Geometry: final body of the model. Coordinates: model frame, mm. A direction names the side the tool comes from. Coordinates: 2 decimals unless noted, no trailing zeros. Loops run counter-clockwise (first coordinate to the right, second up) from the corner with the lowest first, then second, coordinate; pieces in that order, holes last. Notation, with made-up numbers: (-34, 5.5) - (24, 5.5) arc R15 ccw to (24, 24.5) - close; hole circle Ø7 at (28.5, -2). An arc over 180 degrees is marked (long way). Write each question's results on one line, items separated by ' | '. Start each with the question number.
from build123d import *

# Parameters (mm, degrees)
BOSS_EXTRUDE1_DEPTH = 15
SKETCH5_R           = 17
CUT_EXTRUDE3_DEPTH  = 12
SKETCH8_R           = 3.5
CUT_EXTRUDE5_DEPTH  = 3
CUT_EXTRUDE8_DEPTH  = 2
BOSS_EXTRUDE2_DEPTH = 3
BOSS_EXTRUDE3_DEPTH = 3
SKETCH14_R          = 2
SKETCH14_R_2        = 1.65
CUT_EXTRUDE10_DEPTH = 3
SKETCH15_R          = 0.5
SKETCH15_R_2        = 4
SKETCH15_W          = 23.5
SKETCH15_H          = 12.4
CUT_EXTRUDE11_DEPTH = 3
BOSS_EXTRUDE4_DEPTH = 18.1
FILLET2_R           = 5
FILLET3_R           = 1


with BuildPart() as part:
    # Sketch1 → Boss-Extrude1 (new body)
    with BuildSketch(Plane(origin=(0, 0, 0), x_dir=(0, 0, -1), z_dir=(1, 0, 0))):
        with BuildLine():
            Line((0, 20), (80, 20))
            Line((80, 20), (80, -20))
            Line((80, -20), (0, -20))
            ThreePointArc((0, -20), (-20, 0), (0, 20))
        make_face()
    extrude(amount=BOSS_EXTRUDE1_DEPTH)

    # Sketch5 → Cut-Extrude3 (cut)
    with BuildSketch(Plane.ZY):
        Circle(SKETCH5_R)
    extrude(amount=-CUT_EXTRUDE3_DEPTH, mode=Mode.SUBTRACT)

    # Sketch8 → Cut-Extrude5 (cut)
    with BuildSketch(Plane.ZY.offset(-12)):
        Circle(SKETCH8_R)
    extrude(amount=-CUT_EXTRUDE5_DEPTH, mode=Mode.SUBTRACT)

    # Sketch10 → Cut-Extrude8 (cut)
    with BuildSketch(Plane.ZY.offset(-12)):
        with BuildLine():
            Line((-11.740635761, 8.915001197), (-3.490542592, -0.257123349))
            ThreePointArc((-3.490542592, -0.257123349), (-2.474873734, 2.474873734), (0.257123349, 3.490542592))
            Line((0.257123349, 3.490542592), (-8.915001197, 11.740635761))
            ThreePointArc((-8.915001197, 11.740635761), (-11.667842746, 11.667842746), (-11.740635761, 8.915001197))
        make_face()
        with BuildLine():
            Line((11.740635761, -8.915001197), (3.490542592, 0.257123349))
            ThreePointArc((3.490542592, 0.257123349), (3.497634849, 0.12864861), (3.5, 0))
            ThreePointArc((3.5, 0), (2.382233015, -2.564169624), (-0.257123349, -3.490542592))
            Line((-0.257123349, -3.490542592), (8.915001197, -11.740635761))
            ThreePointArc((8.915001197, -11.740635761), (11.667842746, -11.667842746), (11.740635761, -8.915001197))
        make_face()
    extrude(amount=-CUT_EXTRUDE8_DEPTH, mode=Mode.SUBTRACT)

    # Sketch13 → Boss-Extrude3 (add)
    with BuildSketch(Plane(origin=(0, -4.9, 0), x_dir=(1, 0, 0), z_dir=(0, 1, 0))):
        Polygon((-17.5, 80), (32.5, 80), (35.5, 83), (35.5, 103), (30.5, 108), (-15.5, 108), (-20.5, 103), (-20.5, 83), align=None)
    extrude(amount=BOSS_EXTRUDE3_DEPTH)

    # Sketch15 → Cut-Extrude11 (cut)
    with BuildSketch(Plane(origin=(0, -1.9, 0), x_dir=(1, 0, 0), z_dir=(0, 1, 0))):
        with Locations(Location((-16.65, 100, 0), (0, 0, 270))):
            Circle(SKETCH15_R)
        with Locations(Location((11.85, 100, 0), (0, 0, 270))):
            Circle(SKETCH15_R)
        with Locations(Location((22.5, 100, 0), (0, 0, 270))):
            Circle(SKETCH15_R_2)
        with Locations((-2.4, 100)):
            Rectangle(SKETCH15_W, SKETCH15_H)
    extrude(amount=-CUT_EXTRUDE11_DEPTH, mode=Mode.SUBTRACT)



with BuildPart() as body_2:
    # Sketch12 → Boss-Extrude2 (new body)
    with BuildSketch(Plane.XZ.offset(20)):
        Polygon((-17.5, -80), (32.5, -80), (37.5, -85), (37.5, -105), (22, -120.5), (22, -125), (17, -130), (-2, -130), (-7, -125), (-7, -120.5), (-22.5, -105), (-22.5, -85), align=None)
    extrude(amount=-BOSS_EXTRUDE2_DEPTH)

    # Sketch14 → Cut-Extrude10 (cut)
    with BuildSketch(Plane.XZ.offset(20)):
        with Locations(Location((-7.5, -100, 0), (0, 0, 270))):
            Circle(SKETCH14_R)
        with Locations(Location((22.5, -100, 0), (0, 0, 270))):
            Circle(SKETCH14_R_2)
        with Locations(Location((15, -123, 0), (0, 0, 270))):
            Circle(SKETCH14_R_2)
        with Locations(Location((0, -123, 0), (0, 0, 270))):
            Circle(SKETCH14_R_2)
    extrude(amount=-CUT_EXTRUDE10_DEPTH, mode=Mode.SUBTRACT)


with BuildPart() as part_1:
    add(part.part)

    add(body_2.part)  # Boss-Extrude4 merges body 2
    # Sketch16 → Boss-Extrude4 (add)
    with BuildSketch(Plane(origin=(0, -1.9, 0), x_dir=(1, 0, 0), z_dir=(0, 1, 0))):
        Polygon((-17.5, 80), (0, 80), (0, 62.5), align=None)
        Polygon((15, 80), (32.5, 80), (15, 62.5), align=None)
    extrude(amount=-BOSS_EXTRUDE4_DEPTH)

    # Fillet2
    fillet2_edges = [part_1.edges().sort_by_distance(p)[0] for p in [
        (15, -10.95, -62.5),
        (15, -1.9, -71.25),
        (0, -1.9, -71.25),
        (7.5, -1.9, -80),
    ]]
    fillet(fillet2_edges, radius=FILLET2_R)

    # Fillet3
    fillet3_edges = [part_1.edges().sort_by_distance(p)[0] for p in [
        (-7, -20, -122.75),
        (32.5, -10.95, -80),
        (-4.5, -20, -127.5),
        (-20, -17, -82.5),
        (7.5, -20, -130),
        (19.5, -20, -127.5),
        (22, -20, -122.75),
        (29.75, -20, -112.75),
        (37.5, -20, -95),
        (-22.5, -20, -95),
        (-14.75, -20, -112.75),
        (-7, -18.5, -120.5),
        (-7, -18.5, -125),
        (-2, -18.5, -130),
        (35, -17, -82.5),
        (17, -18.5, -130),
        (22, -18.5, -125),
        (22, -18.5, -120.5),
        (37.5, -18.5, -105),
        (37.5, -18.5, -85),
        (-22.5, -18.5, -85),
        (-22.5, -18.5, -105),
        (37.5, -17, -95),
        (29.75, -17, -112.75),
        (22, -17, -122.75),
        (19.5, -17, -127.5),
        (7.5, -17, -130),
        (-4.5, -17, -127.5),
        (-7, -17, -122.75),
        (-14.75, -17, -112.75),
        (-17.5, -10.95, -80),
        (-19, -4.9, -81.5),
        (-20.5, -3.4, -83),
        (34, -4.9, -81.5),
        (35.5, -4.9, -93),
        (35.5, -3.4, -83),
        (33, -4.9, -105.5),
        (35.5, -3.4, -103),
        (7.5, -4.9, -108),
        (30.5, -3.4, -108),
        (-18, -4.9, -105.5),
        (-15.5, -3.4, -108),
        (-20.5, -4.9, -93),
        (-20.5, -3.4, -103),
        (35.5, -1.9, -93),
        (33, -1.9, -105.5),
        (7.5, -1.9, -108),
        (-18, -1.9, -105.5),
        (-20.5, -1.9, -93),
        (-22.5, -17, -95),
    ]]
    fillet(fillet3_edges, radius=FILLET3_R)


solid = part_1.part
1) Section query B-B on y = 14. Output: boundary loops of the cut face in (x, z).
2) Pin query (flat end, axial travel): pin 1 Ø6 at (x, y) = (15.5, -10.5) entering from -Z; pin 2 Ø0.8 at (y, z) = (-18.5, -123) entering from -X; pin 3 Ø14 at (y, z) = (8, -4) entering from -X. Return the tip coordinate at first contact, or that it passes through.
3) Section query C-C on y = 5. Output: boundary loops of the cut face in (x, z).
4) Pull-direction query (Y, two-part tool) for faces 1 (the flat face through (33, -3.4, -105.5)), 2 (the cylindrical face through (29.444, -19.699, -112.653)), 3 (the flat face through (12, 0, 4)), 4 (the flat face through (8, -1.9, -92)); classes: released by +Y, released by -Y, zero draft, split by the parting line, or undercut.
5) Material intervals for line 1 (X direction, y = -2.8, z = -100); line 2 (X direction, y = -18.5, z = -100); line 3 (Y direction, x = -12, z = -84), sorted ascending. Write a range as [from, to].
6) Access query for faces 5 (the flat face through (12.99, -4.39, 7.67)), 6 (the cylindrical face through (-17.82, -4.61, -105.26)), 7 (the flat face through (7, -4.9, -91)), 8 (the cylindrical face through (7, 0, 20)). Directions: +Z, -Z, +X, -X, +Y, -Y. A direction counts if a zero-diameter tool reaches every point of the face in a straight line with its end or side. Return the directions, or none.
7) Section query A-A on z = -73.5. Output: boundary loops of the cut face in (x, y), and give its area (3 significant figures).
Returned:
1) outline: (0, -80) - (15, -80) - (15, 14.28) - (0, 14.28) - (0, 9.64) - (12, 9.64) - (12, -9.64) - (0, -9.64) - close
2) pin 1: stops at z = -80 | pin 2: stops at x = -7 | pin 3: stops at x = 12
3) outline: (0, -80) - (15, -80) - (15, 19.36) - (0, 19.36) - (0, 16.25) - (12, 16.25) - (12, -1.42) - (14, -1.42) - (14, -8.22) - (12, -8.22) - (12, -16.25) - (0, -16.25) - close
4) face 1: zero draft | face 2: released by -Y | face 3: undercut | face 4: released by +Y
5) line 1: x = [-20.49, -17.15], [-16.15, -14.15], [9.35, 11.35], [12.35, 18.5], [26.5, 35.49] | line 2: x = [-22.5, -9.5], [-5.5, 20.85], [24.15, 37.5] | line 3: y = [-20, -17], [-4.9, -1.9]
6) face 5: -X | face 6: -Z, -X | face 7: -Z, +X, -X | face 8: +Z, +X, -X
7) outline: (-11, -20) - (26, -20) - (26, -1.9) - (20, -1.9) arc R5 cw to (15, 3.1) - (15, 20) - (0, 20) - (0, 3.1) arc R5 cw to (-5, -1.9) - (-11, -1.9) - close | area: 1,010 mm²
